```python
from build123d import *

# Parameters (mm, degrees)
PAD_DEPTH            = 18
POCKET_DEPTH         = 6
SKETCH002_R          = 4.25
POCKET001_DEPTH      = 0.001
POCKET001_DEPTH_BACK = 18.001


with BuildPart() as body:
    # Sketch → Pad (new body)
    with BuildSketch(Plane.YZ):
        with BuildLine():
            ThreePointArc((20, 200), (5.857864, 194.142136), (0, 180))
            Line((0, 180), (0, 0))
            Line((0, 0), (60, 0))
            add(Edge.make_bspline(
                [(240, 0), (240, 140), (150, 140), (60, 140), (60, 0)],
                knots=[1.570796, 1.570796, 1.570796, 3.141593, 3.141593, 4.712389, 4.712389, 4.712389], degree=2, weights=[1, 0.707107, 1, 0.707107, 1]))
            Line((240, 0), (300, 0))
            Line((300, 0), (300, 180))
            ThreePointArc((300, 180), (294.142136, 194.142136), (280, 200))
            Line((280, 200), (225, 200))
            Line((225, 200), (75, 200))
            Line((75, 200), (20, 200))
        make_face()
    extrude(amount=PAD_DEPTH)

    # Sketch001 → Pocket (cut)
    with BuildSketch(Plane.YZ.offset(18)):
        Polygon((28, 92), (28, 162), (290, 162), (290, 180), (10, 180), (10, 92), align=None)
    extrude(amount=-POCKET_DEPTH, mode=Mode.SUBTRACT)

    # Sketch002 → Pocket001 (cut, two sides)
    with BuildSketch(Plane.YZ) as pocket001_sk:
        with Locations((19, 137)):
            Circle(SKETCH002_R)
        with Locations((19, 117)):
            Circle(SKETCH002_R)
        with Locations((35, 171)):
            Circle(SKETCH002_R)
        with Locations((265, 171)):
            Circle(SKETCH002_R)
    extrude(amount=-POCKET001_DEPTH, mode=Mode.SUBTRACT)
    extrude(pocket001_sk.sketch, amount=POCKET001_DEPTH_BACK, mode=Mode.SUBTRACT)


with BuildPart() as part_mirroring:
    # Part__Mirroring: instance of Body
    add(body.part.mirror(Plane(origin=(0, 0, 0), x_dir=(1, 0, 0), z_dir=(0, 1, 0))))


solid = part_mirroring.part
```
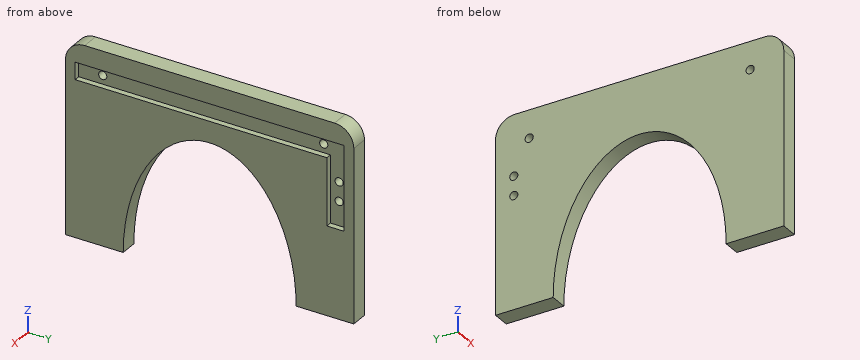
Verification items for the finished model (mm, model axes). Coordinates: 2 decimals unless noted, no trailing zeros. Loops run counter-clockwise (first coordinate to the right, second up) from the corner with the lowest first, then second, coordinate; pieces in that order, holes last. Notation, with made-up numbers: (87, 52.25) -> (92, 52.25) arc R19 cw to (92, 83.25) -> close; hole circle Ø11 at (57.25, 0). An arc over 180 degrees is marked (long way). Put each result on its own line as item: value.
1. Section check B-B, the plane y = -49.5. Record the boundary of the cut face in (x, z), then the cut area to 3 significant figures.
Result set:
outline: (0, 0) -> (18, 0) -> (18, 162) -> (12, 162) -> (12, 180) -> (18, 180) -> (18, 200) -> (0, 200) -> close
area: 3,490 mm^2
2. Thickness scan on line 1 (Z direction, x = 8, y = -19); line 2 (Y direction, x = 9, z = 171); line 3 (Z direction, x = 11.5, y = -21). Record the ranges inside material, lowest first.
Result set:
line 1: z = 0 to 112.75, 121.25 to 132.75, 141.25 to 199.97
line 2: y = -300 to -269.25, -260.75 to -39.25, -30.75 to 0
line 3: z = 0 to 113.25, 120.75 to 133.25, 140.75 to 200
3. Gauge pin test, flat ends, axial feed: P1, Ø6, axis at x = 15.5, y = -183.5, coming from the -Z side; P2, Ø3, axis at x = 14, y = -190.5, coming from the -Z side; P3, Ø2, axis at x = 2.5, y = -122, coming from the -Z side. Record the tip position at first contact, or that the pin passes through.
Result set:
P1: stops at z = 127.97
P2: stops at z = 123.82
P3: stops at z = 132.53
4. Section check C-C, the plane y = -265. Record the boundary of the cut face in (x, z).
Result set:
outline: (0, 0) -> (18, 0) -> (18, 162) -> (12, 162) -> (12, 166.75) -> (0, 166.75) -> close; (0, 175.25) -> (12, 175.25) -> (12, 180) -> (18, 180) -> (18, 200) -> (0, 200) -> close
5. Section check D-D, the plane x = 5.75. Give the number of separate pieces and of enclosed holes in the cut face, then the cut area to 3 significant figures.
Result set:
separate pieces: 1
enclosed holes: 4
area: 39,800 mm^2
6. Section check A-A, the plane z = 171. Record the boundary of the cut face in (x, y), then the cut area to 3 significant figures.
Result set:
outline: (0, -300) -> (18, -300) -> (18, -290) -> (12, -290) -> (12, -269.25) -> (0, -269.25) -> close; (0, -260.75) -> (12, -260.75) -> (12, -39.25) -> (0, -39.25) -> close; (0, -30.75) -> (12, -30.75) -> (12, -10) -> (18, -10) -> (18, 0) -> (0, 0) -> close
area: 3,520 mm^2
